Geometry check sheet. Reference: the model listing, model coordinates, mm. A direction names the side the tool comes from. Coordinates: 2 decimals unless noted, no trailing zeros. Write each loop counter-clockwise with the first axis right and the second up, starting at its lowest first coordinate (ties: lowest second). Pieces come first, ordered by that corner, then holes. Notation, with made-up numbers: (52, 13) -> (111, 13) arc R27 cw to (111, 36) -> close; hole circle Ø2 at (79, 24.5). An arc over 180 degrees is marked (long way). Use a Markdown table: item, result.
```python
from build123d import *

# Parameters (mm, degrees)
SKETCH1_W               = 93.5
SKETCH1_H               = 45
BOSS_EXTRUDE1_DEPTH     = 5
SKETCH2_R               = 1.75
CUT_EXTRUDE1_DEPTH      = 1
CUT_EXTRUDE1_DEPTH_BACK = 6
SKETCH3_R               = 2.9
CUT_EXTRUDE2_DEPTH      = 1
CUT_EXTRUDE2_DEPTH_BACK = 3


with BuildPart() as part:
    # Sketch1 → Boss-Extrude1 (new body)
    with BuildSketch(Plane(origin=(0, 0, 0), x_dir=(1, 0, 0), z_dir=(0, 1, 0))):
        Rectangle(SKETCH1_W, SKETCH1_H)
    extrude(amount=BOSS_EXTRUDE1_DEPTH)

    # Sketch2 → Cut-Extrude1 (cut, two sides)
    with BuildSketch(Plane(origin=(0, 5, 0), x_dir=(1, 0, 0), z_dir=(0, 1, 0))) as cut_extrude1_sk:
        with Locations((-9.75, -16.5)):
            Circle(SKETCH2_R)
        with Locations((-9.75, 16.5)):
            Circle(SKETCH2_R)
        with Locations((9.75, -16.5)):
            Circle(SKETCH2_R)
        with Locations((9.75, 16.5)):
            Circle(SKETCH2_R)
    extrude(amount=CUT_EXTRUDE1_DEPTH, mode=Mode.SUBTRACT)
    extrude(cut_extrude1_sk.sketch, amount=-CUT_EXTRUDE1_DEPTH_BACK, mode=Mode.SUBTRACT)

    # Sketch3 → Cut-Extrude2 (cut, two sides)
    with BuildSketch(Plane(origin=(0, 5, 0), x_dir=(1, 0, 0), z_dir=(0, 1, 0))) as cut_extrude2_sk:
        with Locations((-9.75, 16.5)):
            Circle(SKETCH3_R)
        with Locations((9.75, 16.5)):
            Circle(SKETCH3_R)
        with Locations((9.75, -16.5)):
            Circle(SKETCH3_R)
        with Locations((-9.75, -16.5)):
            Circle(SKETCH3_R)
    extrude(amount=CUT_EXTRUDE2_DEPTH, mode=Mode.SUBTRACT)
    extrude(cut_extrude2_sk.sketch, amount=-CUT_EXTRUDE2_DEPTH_BACK, mode=Mode.SUBTRACT)


solid = part.part
```
Item 1: Section check B-B on y = 4. Record the boundary of the cut face in (x, z), then the cut area to 3 significant figures.
Answer block:
| item | result |
|---|---|
| outline | (-46.75, -22.5) -> (46.75, -22.5) -> (46.75, 22.5) -> (-46.75, 22.5) -> close; hole circle Ø5.8 at (-9.75, -16.5); hole circle Ø5.8 at (-9.75, 16.5); hole circle Ø5.8 at (9.75, -16.5); hole circle Ø5.8 at (9.75, 16.5) |
| area | 4,100 mm^2 |
Item 2: Tool access check on faces 4 (the flat face through (-1, 0, 0)), 5 (the cylindrical face through (7.449, 3.521, -14.735)). Record the directions out of +Z, -Z, +X, -X, +Y, -Y that give a thin tool (end or side, any length) a straight path to the whole face; none if there is none.
Answer block:
| item | result |
|---|---|
| face 4 | +Z, -Z, +X, -X, -Y |
| face 5 | +Y |
Item 3: Section check A-A on x = 9.75. Record the boundary of the cut face in (y, z).
Answer block:
| item | result |
|---|---|
| outline | (0, -22.5) -> (5, -22.5) -> (5, -19.4) -> (2, -19.4) -> (2, -18.25) -> (0, -18.25) -> close; (0, -14.75) -> (2, -14.75) -> (2, -13.6) -> (5, -13.6) -> (5, 13.6) -> (2, 13.6) -> (2, 14.75) -> (0, 14.75) -> close; (0, 18.25) -> (2, 18.25) -> (2, 19.4) -> (5, 19.4) -> (5, 22.5) -> (0, 22.5) -> close |
Item 4: Mould release check, pull along Z, two halves, no side actions. Record for faces 1 (the flat face through (-1, 2, -22.5)), 2 (the cylindrical face through (-9.978, 1.014, -18.235)), 3 (the flat face through (-46.75, 2, 0)): +Z half, -Z half, draft (parallel to the pull), parting line (faces both ways), or undercut.
Answer block:
| item | result |
|---|---|
| face 1 | -Z half |
| face 2 | undercut |
| face 3 | draft |
Item 5: Depth check by flat-ended pin: P1, Ø4.5, axis at x = 9.75, z = -16.5, coming from the +Y side; P2, Ø3, axis at x = 9.75, z = -16.5, coming from the +Y side. Enter the tip coordinate at first touch or a pass-through.
Answer block:
| item | result |
|---|---|
| P1 | stops at y = 2 |
| P2 | passes through |
Item 6: Thickness scan on L1, parallel to Z at x = 9.75, y = 2.7; L2, parallel to X at y = 0.5, z = -16.5; L3, parallel to Z at x = 9.75, y = 1.05. Record the ranges inside material, lowest first. Write a range as [from, to].
Answer block:
| item | result |
|---|---|
| L1 | z = [-22.5, -19.4], [-13.6, 13.6], [19.4, 22.5] |
| L2 | x = [-46.75, -11.5], [-8, 8], [11.5, 46.75] |
| L3 | z = [-22.5, -18.25], [-14.75, 14.75], [18.25, 22.5] |
